```python
from build123d import *

# Parameters (mm, degrees)
SKETCH2_W               = 50.634745493
SKETCH2_H               = 13.07277583
CUT_EXTRUDE1_DEPTH      = 5.0000001
CUT_EXTRUDE1_DEPTH_BACK = 5.0000001
SKETCH3_R               = 1
CUT_EXTRUDE2_DEPTH      = 5.0000001
SKETCH4_R               = 2.1
CUT_EXTRUDE3_DEPTH      = 4.0000001
SKETCH5_R               = 1.5
CUT_EXTRUDE4_DEPTH      = 5.0000001
CUT_EXTRUDE5_DEPTH      = 1.0000001
CUT_EXTRUDE5_DEPTH_BACK = 5.0000001


with BuildPart() as part:
    # Sketch1 → Revolve1 (revolve)
    with BuildSketch(Plane.XY):
        with BuildLine():
            Line((-14, 0), (14, 0))
            add(Edge.make_bspline(
                [(14, 0), (14, 4), (0, 4), (-14, 4), (-14, 0)],
                knots=[0, 0, 0, 1.570796327, 1.570796327, 3.141592654, 3.141592654, 3.141592654], degree=2, weights=[1, 0.707106781, 1, 0.707106781, 1]))
        make_face()
    revolve(axis=Axis((-14, 0, 0), (1, 0, 0)))

    # Sketch2 → Cut-Extrude1 (cut, two sides)
    with BuildSketch(Plane.XY) as cut_extrude1_sk:
        with Locations((-1.598405816, -6.536387915)):
            Rectangle(SKETCH2_W, SKETCH2_H)
    extrude(amount=CUT_EXTRUDE1_DEPTH, mode=Mode.SUBTRACT)
    extrude(cut_extrude1_sk.sketch, amount=-CUT_EXTRUDE1_DEPTH_BACK, mode=Mode.SUBTRACT)

    # Sketch3 → Cut-Extrude2 (cut, through all)
    with BuildSketch(Plane.XZ):
        with Locations((-10.5, 0)):
            Circle(SKETCH3_R)
        with Locations((-2.5, 0)):
            Circle(SKETCH3_R)
    extrude(amount=-CUT_EXTRUDE2_DEPTH, mode=Mode.SUBTRACT)

    # Sketch4 → Cut-Extrude3 (cut, through all)
    with BuildSketch(Plane(origin=(0, 1, 0), x_dir=(-1, 0, 0), z_dir=(0, -1, 0))):
        with Locations((10.5, 0)):
            Circle(SKETCH4_R)
        with Locations((2.5, 0)):
            Circle(SKETCH4_R)
    extrude(amount=-CUT_EXTRUDE3_DEPTH, mode=Mode.SUBTRACT)

    # Sketch5 → Cut-Extrude4 (cut, through all)
    with BuildSketch(Plane.XZ):
        with Locations((2, -0.36)):
            Circle(SKETCH5_R)
    extrude(amount=-CUT_EXTRUDE4_DEPTH, mode=Mode.SUBTRACT)

    # Sketch6 → Cut-Extrude5 (cut, two sides)
    with BuildSketch(Plane.XZ) as cut_extrude5_sk:
        with BuildLine():
            Line((6.957274385, 3.471120893), (2, 0))
            Line((2, 0), (4.642362064, -3.773684114))
            add(Edge.make_bspline(
                [(4.642362064, -3.773684114), (14, -2.833952984), (14, 0)],
                knots=[5.050385136, 5.050385136, 5.050385136, 6.283185307, 6.283185307, 6.283185307], degree=2, weights=[1, 0.815964855, 1]))
            add(Edge.make_bspline(
                [(14, 0), (14, 2.318798314), (6.957274385, 3.471120893)],
                knots=[0, 0, 0, 1.05071793, 1.05071793, 1.05071793], degree=2, weights=[1, 0.865143968, 1]))
        make_face()
    extrude(amount=CUT_EXTRUDE5_DEPTH, mode=Mode.SUBTRACT)
    extrude(cut_extrude5_sk.sketch, amount=-CUT_EXTRUDE5_DEPTH_BACK, mode=Mode.SUBTRACT)


solid = part.part
```
Geometry: final body of the model. Coordinates: model frame, mm. A direction names the side the tool comes from. Round coordinates to 2 decimals unless told otherwise and drop trailing zeros. One line per item, written item: value.
(1) Line query: probe 1 along X at (y, z) = (2.65, -0.25); probe 2 along Y at (x, z) = (-9, 0); probe 3 along Z at (x, y) = (2, 2.8). Output: solid intervals per line, ascending. Write a range as [from, to].
Result sheet:
probe 1: [-8.41, -4.59], [-0.41, 0.5]
probe 2: [0, 1]
probe 3: [-2.8, -1.86], [1.14, 2.8]
(2) Pull-direction query (Z, two-part tool) for faces 1 (the flat face through (-4, 0, 0)), 2 (the flat face through (3.64, 1.38, -2.34)), 3 (the cylindrical face through (-11.3, 0.5, -0.6)); classes: pulls with the +Z half, pulls with the -Z half, needs draft (parallel to the pull), parting line crosses it, or undercut.
Result sheet:
face 1: needs draft
face 2: undercut
face 3: undercut
(3) Reachability of faces 4 (the cylindrical face through (0.5, 2, -0.3)), 5 (the cylindrical face through (-8.4, 1.84, -0.09)), 6 (the flat face through (4.588, 1.465, 1.812)) from +Z, -Z, +X, -X, +Y, -Y: full face, straight path, thin tool, end or side. Return the list, or none.
Result sheet:
face 4: +Y, -Y
face 5: +Y
face 6: +X, +Y, -Y
(4) Cut plane A-A (z = 0). Give the number of separate pieces and of enclosed holes in the cut face, and give its area (3 significant figures).
Result sheet:
separate pieces: 3
enclosed holes: 0
area: 23.2 mm2
(5) Pin query (flat end, axial travel): P1, Ø1, axis at y = 1.5, z = -0.5, coming from the +X side; P2, Ø4, axis at x = -2.5, z = 0, coming from the -Y side; P3, Ø1.5, axis at x = -4, z = 3, coming from the +Y side; P4, Ø1.8, axis at x = -10.5, z = 0, coming from the -Y side. Return the tip coordinate at first contact, or that it passes through.
Result sheet:
P1: x = 0.64
P2: y = 0
P3: y = 3.11
P4: through
